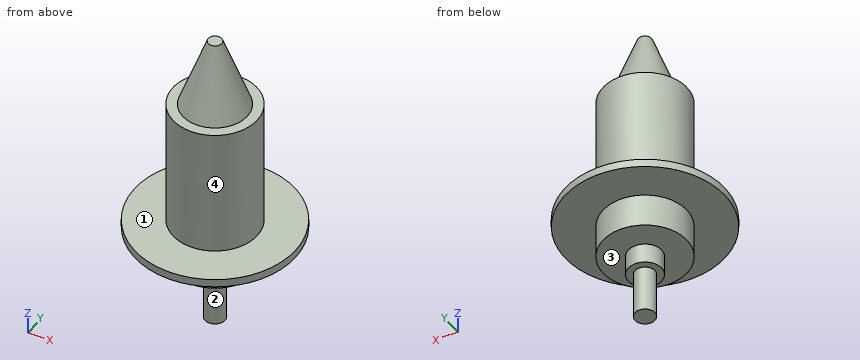
```python
from build123d import *

# Parameters (mm, degrees)
CYLINDER002_R     = 2.5
CYLINDER002_DEPTH = 3
CYLINDER001_R     = 12
CYLINDER001_DEPTH = 1.2
CYLINDER_R        = 6.3
CYLINDER_DEPTH    = 25.5
CYLINDER003_R     = 1.5
CYLINDER003_DEPTH = 10


with BuildPart() as cylinder002:
    # Cylinder002 → Cylinder002 (new body)
    with BuildSketch(Plane.XY.offset(-3)):
        Circle(CYLINDER002_R)
    extrude(amount=CYLINDER002_DEPTH)


with BuildPart() as cylinder001:
    # Cylinder001 → Cylinder001 (new body)
    with BuildSketch(Plane.XY.offset(5)):
        Circle(CYLINDER001_R)
    extrude(amount=CYLINDER001_DEPTH)


with BuildPart() as cylinder:
    # Cylinder → Cylinder (new body)
    with BuildSketch(Plane.XY):
        Circle(CYLINDER_R)
    extrude(amount=CYLINDER_DEPTH)


with BuildPart() as cylinder003:
    # Cylinder003 → Cylinder003 (new body)
    with BuildSketch(Plane.XY.offset(-10)):
        Circle(CYLINDER003_R)
    extrude(amount=CYLINDER003_DEPTH)


with BuildPart() as assembly:
    # Cone → Cone (revolve)
    with BuildSketch(Plane(origin=(0, 0, 25), x_dir=(1, 0, 0), z_dir=(0, -1, 0))):
        Polygon((0, 0), (5, 0), (1, 11), (0, 11), align=None)
    revolve(axis=Axis((0, 0, 25), (0, 0, 1)))

    # Fusion: union Cylinder002, Cylinder001, Cylinder, Cylinder003
    add(cylinder002.part)
    add(cylinder001.part)
    add(cylinder.part)
    add(cylinder003.part)


solid = assembly.part
```
Read the model definition and answer for the solid it produces. Units are mm, in the model's axes. Face numbers are marked on the shaded views. A direction names the side the tool comes from. Round coordinates to 2 decimals unless told otherwise and drop trailing zeros. Write each loop counter-clockwise with the first axis right and the second up, starting at its lowest first coordinate (ties: lowest second). Pieces come first, ordered by that corner, then holes. Notation, with made-up numbers: (-2, 80) - (46, 80) arc R16 ccw to (46, 89) - close; hole circle Ø3 at (-19.5, -23.5). An arc over 180 degrees is marked (long way). One line per item, written item: value.
Q1. Which of the six approach directions +Z, -Z, +X, -X, +Y, -Y give full straight-line access (tool end or side, diameter ignored) to the marked faces 1 and 2?
The answers:
face 1: +Z
face 2: -Z
Q2. For a pull along Y with two mould halves and no side action, classify the marked faces 3 and 4 as pulls with the +Y half, pulls with the -Y half, needs draft (parallel to the pull), parting line crosses it, or undercut.
The answers:
face 3: needs draft
face 4: parting line crosses it
Q3. Find section D-D (y = -10.25). Determine the outline of the cut face in (x, z), and give its area (3 significant figures).
The answers:
outline: (-6.24, 5) - (6.24, 5) - (6.24, 6.2) - (-6.24, 6.2) - close
area: 15.0 mm2
Q4. Straight lines are drawn through the part: line 1 (Z direction, x = -7, y = -6); line 2 (Z direction, x = -3.5, y = 3.5); line 3 (Y direction, x = 0.25, z = 24.5). For each, find the intervals that lie inside material, in ascending order. Write a range as from..to.
The answers:
line 1: z = 5..6.2
line 2: z = 0..25.5
line 3: y = -6.3..6.3
Q5. Find section A-A (y = 0). Determine the outline of the cut face in (x, z).
The answers:
outline: (-12, 5) - (-6.3, 5) - (-6.3, 0) - (-2.5, 0) - (-2.5, -3) - (-1.5, -3) - (-1.5, -10) - (1.5, -10) - (1.5, -3) - (2.5, -3) - (2.5, 0) - (6.3, 0) - (6.3, 5) - (12, 5) - (12, 6.2) - (6.3, 6.2) - (6.3, 25.5) - (4.82, 25.5) - (1, 36) - (-1, 36) - (-4.82, 25.5) - (-6.3, 25.5) - (-6.3, 6.2) - (-12, 6.2) - close
Q6. Each of these flat-tipped pins is pushed along its axis until it touches: P1, Ø5, axis at x = 8, z = 9.5, coming from the +Y side; P2, Ø8, axis at x = -2, z = 17, coming from the -Y side; P3, Ø1, axis at x = -0.5, z = 17.5, coming from the +Y side; P4, Ø1.5, axis at y = 8.5, z = 17.5, coming from the -X side. Where does it stop, or does it pass through?
The answers:
P1: stops at y = 3.07
P2: stops at y = -6.3
P3: stops at y = 6.3
P4: passes through
Q7. Find section C-C (z = 22). Determine the outline of the cut face in (x, y), and give its area (3 significant figures).
The answers:
outline: circle Ø12.6 at (0, 0)
area: 125 mm2
